Input: part model. Units: mm. Frame: model coordinates. Face numbers are marked on the shaded views. A direction names the side the tool comes from. Give positions to 0.01 mm unless a question says otherwise; leave off trailing zeros. Loops run counter-clockwise (first coordinate to the right, second up) from the corner with the lowest first, then second, coordinate; pieces in that order, holes last. Notation, with made-up numbers: M 86.5,-11.5 L 113.5,-11.5 A12 cw 113.5,6.5 Z; hole C 88,18.25 d7. An arc over 180 degrees is marked long. Use a Markdown table: item, result. Add a question column.
from build123d import *

# Parameters (mm, degrees)
F0_W     = 50
F0_H     = 1.4
F0_H_2   = 9.33334
F0_H_3   = 9.33333
F0_W_2   = 2
F1_DEPTH = 2
F2_DEPTH = 12.2
F3_DEPTH = 4.4


with BuildPart() as f1:
    # F0 (on Top) → F1 (new body)
    with BuildSketch(Plane.XY):
        with BuildLine():
            ThreePointArc((21.8201372772, -22.06666), (27.3605822843, -24.3541997855), (25.0540951786, -18.8216157258))
            Line((25.0540951786, -18.8216157258), (25.0540951786, -20.06666))
            Line((25.0540951786, -20.06666), (25.0540951786, -20.46666))
            ThreePointArc((25.0540951786, -20.46666), (26.1854660285, -20.9352891501), (26.6540951786, -22.06666))
            ThreePointArc((26.6540951786, -22.06666), (25.0540951786, -23.66666), (23.4540951786, -22.06666))
            Line((23.4540951786, -22.06666), (23.0540951786, -22.06666))
            Line((23.0540951786, -22.06666), (21.8201372772, -22.06666))
        make_face()
        with Locations((-1.9459048214, 0.7)):
            Rectangle(F0_W, F0_H)
        with BuildLine():
            Line((-26.9459048214, 12.73334), (-27.3459048214, 12.73334))
            ThreePointArc((-27.3459048214, 12.73334), (-27.8145339715, 11.6019691501), (-28.9459048214, 11.13334))
            Line((-28.9459048214, 11.13334), (-28.9459048214, 10.73334))
            Line((-28.9459048214, 10.73334), (-26.9459048214, 10.73334))
            Line((-26.9459048214, 10.73334), (-26.9459048214, 12.73334))
        make_face()
        with BuildLine():
            Line((-26.9459048214, -22.06666), (-26.9459048214, -20.06666))
            Line((-26.9459048214, -20.06666), (-28.9459048214, -20.06666))
            Line((-28.9459048214, -20.06666), (-28.9459048214, -20.46666))
            ThreePointArc((-28.9459048214, -20.46666), (-27.8145339715, -20.9352891501), (-27.3459048214, -22.06666))
            Line((-27.3459048214, -22.06666), (-26.9459048214, -22.06666))
        make_face()
        with BuildLine():
            Line((23.0540951786, 12.73334), (23.0540951786, 10.73334))
            Line((23.0540951786, 10.73334), (25.0540951786, 10.73334))
            Line((25.0540951786, 10.73334), (25.0540951786, 11.1939641141))
            ThreePointArc((25.0540951786, 11.1939641141), (23.9822411075, 11.6614859288), (23.5147192927, 12.73334))
            Line((23.5147192927, 12.73334), (23.0540951786, 12.73334))
        make_face()
        with Locations((-1.9459048214, 6.06667)):
            Rectangle(F0_W, F0_H_2)
        Polygon((-26.9459048214, 10.73334), (-28.9459048214, 10.73334), (-28.9459048214, 9.7067784518), (-28.9459048214, 1.4), (-26.9459048214, 1.4), align=None)
        with Locations((-1.9459048214, -4.666665)):
            Rectangle(F0_W, F0_H_3)
        with BuildLine():
            ThreePointArc((25.0540951786, 9.4220731407), (27.3739572404, 15.169460212), (21.67487517, 12.73334))
            Line((21.67487517, 12.73334), (23.0540951786, 12.73334))
            Line((23.0540951786, 12.73334), (23.5147192927, 12.73334))
            ThreePointArc((23.5147192927, 12.73334), (25.0838484178, 14.3925799209), (26.7136119574, 12.7928567787))
            ThreePointArc((26.7136119574, 12.7928567787), (26.2237410386, 11.6406356962), (25.0540951786, 11.1939641141))
            Line((25.0540951786, 11.1939641141), (25.0540951786, 10.73334))
            Line((25.0540951786, 10.73334), (25.0540951786, 9.4220731407))
        make_face()
        with Locations((24.0540951786, -10.03333)):
            Rectangle(F0_W_2, F0_H)
        with BuildLine():
            ThreePointArc((-28.9459048214, 11.13334), (-30.0772756713, 13.8647108499), (-27.3459048214, 12.73334))
            Line((-27.3459048214, 12.73334), (-26.9459048214, 12.73334))
            Line((-26.9459048214, 12.73334), (-26.0620750487, 12.73334))
            ThreePointArc((-26.0620750487, 12.73334), (-31.1388180647, 14.6834699023), (-28.9459048214, 9.7067784518))
            Line((-28.9459048214, 9.7067784518), (-28.9459048214, 10.73334))
            Line((-28.9459048214, 10.73334), (-28.9459048214, 11.13334))
        make_face()
        with BuildLine():
            Line((-28.9459048214, -20.06666), (-28.9459048214, -19.0631560981))
            ThreePointArc((-28.9459048214, -19.0631560981), (-31.0781165452, -24.1453706629), (-25.9737856686, -22.06666))
            Line((-25.9737856686, -22.06666), (-26.9459048214, -22.06666))
            Line((-26.9459048214, -22.06666), (-27.3459048214, -22.06666))
            ThreePointArc((-27.3459048214, -22.06666), (-30.0772756713, -23.1980308499), (-28.9459048214, -20.46666))
            Line((-28.9459048214, -20.46666), (-28.9459048214, -20.06666))
        make_face()
        Polygon((-26.0620750487, 12.73334), (-26.9459048214, 12.73334), (-26.9459048214, 10.73334), (23.0540951786, 10.73334), (23.0540951786, 12.73334), (21.67487517, 12.73334), align=None)
        Polygon((23.0540951786, -20.06666), (-26.9459048214, -20.06666), (-26.9459048214, -22.06666), (-25.9737856686, -22.06666), (21.8201372772, -22.06666), (23.0540951786, -22.06666), align=None)
        with Locations((-27.9459048214, 0.7)):
            Rectangle(F0_W_2, F0_H)
        with Locations((24.0540951786, 0.7)):
            Rectangle(F0_W_2, F0_H)
        with Locations((-27.9459048214, -4.666665)):
            Rectangle(F0_W_2, F0_H_3)
        with Locations((24.0540951786, -4.666665)):
            Rectangle(F0_W_2, F0_H_3)
        with Locations((-27.9459048214, -10.03333)):
            Rectangle(F0_W_2, F0_H)
        with Locations((-1.9459048214, -15.399995)):
            Rectangle(F0_W, F0_H_3)
        with BuildLine():
            Line((25.0540951786, -20.06666), (23.0540951786, -20.06666))
            Line((23.0540951786, -20.06666), (23.0540951786, -22.06666))
            Line((23.0540951786, -22.06666), (23.4540951786, -22.06666))
            ThreePointArc((23.4540951786, -22.06666), (23.9227243287, -20.9352891501), (25.0540951786, -20.46666))
            Line((25.0540951786, -20.46666), (25.0540951786, -20.06666))
        make_face()
        Polygon((-26.9459048214, -20.06666), (-26.9459048214, -10.73333), (-28.9459048214, -10.73333), (-28.9459048214, -19.0631560981), (-28.9459048214, -20.06666), align=None)
        Polygon((25.0540951786, 10.73334), (23.0540951786, 10.73334), (23.0540951786, 1.4), (25.0540951786, 1.4), (25.0540951786, 9.4220731407), align=None)
        with Locations((-1.9459048214, -10.03333)):
            Rectangle(F0_W, F0_H)
        Polygon((25.0540951786, -10.73333), (23.0540951786, -10.73333), (23.0540951786, -20.06666), (25.0540951786, -20.06666), (25.0540951786, -18.8216157258), align=None)
    extrude(amount=F1_DEPTH)

    # F0 (on Top) → F2 (join)
    with BuildSketch(Plane.XY):
        Polygon((-26.0620750487, 12.73334), (-26.9459048214, 12.73334), (-26.9459048214, 10.73334), (23.0540951786, 10.73334), (23.0540951786, 12.73334), (21.67487517, 12.73334), align=None)
        Polygon((-26.9459048214, 10.73334), (-28.9459048214, 10.73334), (-28.9459048214, 9.7067784518), (-28.9459048214, 1.4), (-26.9459048214, 1.4), align=None)
        with Locations((-27.9459048214, -4.666665)):
            Rectangle(F0_W_2, F0_H_3)
        Polygon((-26.9459048214, -20.06666), (-26.9459048214, -10.73333), (-28.9459048214, -10.73333), (-28.9459048214, -19.0631560981), (-28.9459048214, -20.06666), align=None)
        Polygon((23.0540951786, -20.06666), (-26.9459048214, -20.06666), (-26.9459048214, -22.06666), (-25.9737856686, -22.06666), (21.8201372772, -22.06666), (23.0540951786, -22.06666), align=None)
        Polygon((25.0540951786, -10.73333), (23.0540951786, -10.73333), (23.0540951786, -20.06666), (25.0540951786, -20.06666), (25.0540951786, -18.8216157258), align=None)
        with Locations((24.0540951786, -4.666665)):
            Rectangle(F0_W_2, F0_H_3)
        with Locations((24.0540951786, -10.03333)):
            Rectangle(F0_W_2, F0_H)
        with Locations((-27.9459048214, -10.03333)):
            Rectangle(F0_W_2, F0_H)
        Polygon((25.0540951786, 10.73334), (23.0540951786, 10.73334), (23.0540951786, 1.4), (25.0540951786, 1.4), (25.0540951786, 9.4220731407), align=None)
        with Locations((24.0540951786, 0.7)):
            Rectangle(F0_W_2, F0_H)
        with Locations((-27.9459048214, 0.7)):
            Rectangle(F0_W_2, F0_H)
        with BuildLine():
            ThreePointArc((25.0540951786, 9.4220731407), (27.3739572404, 15.169460212), (21.67487517, 12.73334))
            Line((21.67487517, 12.73334), (23.0540951786, 12.73334))
            Line((23.0540951786, 12.73334), (23.5147192927, 12.73334))
            ThreePointArc((23.5147192927, 12.73334), (25.0838484178, 14.3925799209), (26.7136119574, 12.7928567787))
            ThreePointArc((26.7136119574, 12.7928567787), (26.2237410386, 11.6406356962), (25.0540951786, 11.1939641141))
            Line((25.0540951786, 11.1939641141), (25.0540951786, 10.73334))
            Line((25.0540951786, 10.73334), (25.0540951786, 9.4220731407))
        make_face()
        with BuildLine():
            ThreePointArc((21.8201372772, -22.06666), (27.3605822843, -24.3541997855), (25.0540951786, -18.8216157258))
            Line((25.0540951786, -18.8216157258), (25.0540951786, -20.06666))
            Line((25.0540951786, -20.06666), (25.0540951786, -20.46666))
            ThreePointArc((25.0540951786, -20.46666), (26.1854660285, -20.9352891501), (26.6540951786, -22.06666))
            ThreePointArc((26.6540951786, -22.06666), (25.0540951786, -23.66666), (23.4540951786, -22.06666))
            Line((23.4540951786, -22.06666), (23.0540951786, -22.06666))
            Line((23.0540951786, -22.06666), (21.8201372772, -22.06666))
        make_face()
        with BuildLine():
            Line((25.0540951786, -20.06666), (23.0540951786, -20.06666))
            Line((23.0540951786, -20.06666), (23.0540951786, -22.06666))
            Line((23.0540951786, -22.06666), (23.4540951786, -22.06666))
            ThreePointArc((23.4540951786, -22.06666), (23.9227243287, -20.9352891501), (25.0540951786, -20.46666))
            Line((25.0540951786, -20.46666), (25.0540951786, -20.06666))
        make_face()
        with BuildLine():
            Line((23.0540951786, 12.73334), (23.0540951786, 10.73334))
            Line((23.0540951786, 10.73334), (25.0540951786, 10.73334))
            Line((25.0540951786, 10.73334), (25.0540951786, 11.1939641141))
            ThreePointArc((25.0540951786, 11.1939641141), (23.9822411075, 11.6614859288), (23.5147192927, 12.73334))
            Line((23.5147192927, 12.73334), (23.0540951786, 12.73334))
        make_face()
        with BuildLine():
            Line((-26.9459048214, -22.06666), (-26.9459048214, -20.06666))
            Line((-26.9459048214, -20.06666), (-28.9459048214, -20.06666))
            Line((-28.9459048214, -20.06666), (-28.9459048214, -20.46666))
            ThreePointArc((-28.9459048214, -20.46666), (-27.8145339715, -20.9352891501), (-27.3459048214, -22.06666))
            Line((-27.3459048214, -22.06666), (-26.9459048214, -22.06666))
        make_face()
        with BuildLine():
            Line((-28.9459048214, -20.06666), (-28.9459048214, -19.0631560981))
            ThreePointArc((-28.9459048214, -19.0631560981), (-31.0781165452, -24.1453706629), (-25.9737856686, -22.06666))
            Line((-25.9737856686, -22.06666), (-26.9459048214, -22.06666))
            Line((-26.9459048214, -22.06666), (-27.3459048214, -22.06666))
            ThreePointArc((-27.3459048214, -22.06666), (-30.0772756713, -23.1980308499), (-28.9459048214, -20.46666))
            Line((-28.9459048214, -20.46666), (-28.9459048214, -20.06666))
        make_face()
        with BuildLine():
            ThreePointArc((-28.9459048214, 11.13334), (-30.0772756713, 13.8647108499), (-27.3459048214, 12.73334))
            Line((-27.3459048214, 12.73334), (-26.9459048214, 12.73334))
            Line((-26.9459048214, 12.73334), (-26.0620750487, 12.73334))
            ThreePointArc((-26.0620750487, 12.73334), (-31.1388180647, 14.6834699023), (-28.9459048214, 9.7067784518))
            Line((-28.9459048214, 9.7067784518), (-28.9459048214, 10.73334))
            Line((-28.9459048214, 10.73334), (-28.9459048214, 11.13334))
        make_face()
        with BuildLine():
            Line((-26.9459048214, 12.73334), (-27.3459048214, 12.73334))
            ThreePointArc((-27.3459048214, 12.73334), (-27.8145339715, 11.6019691501), (-28.9459048214, 11.13334))
            Line((-28.9459048214, 11.13334), (-28.9459048214, 10.73334))
            Line((-28.9459048214, 10.73334), (-26.9459048214, 10.73334))
            Line((-26.9459048214, 10.73334), (-26.9459048214, 12.73334))
        make_face()
    extrude(amount=F2_DEPTH)

    # F0 (on Top) → F3 (join)
    with BuildSketch(Plane.XY):
        with Locations((-1.9459048214, 0.7)):
            Rectangle(F0_W, F0_H)
        with Locations((-1.9459048214, -10.03333)):
            Rectangle(F0_W, F0_H)
    extrude(amount=F3_DEPTH)


solid = f1.part
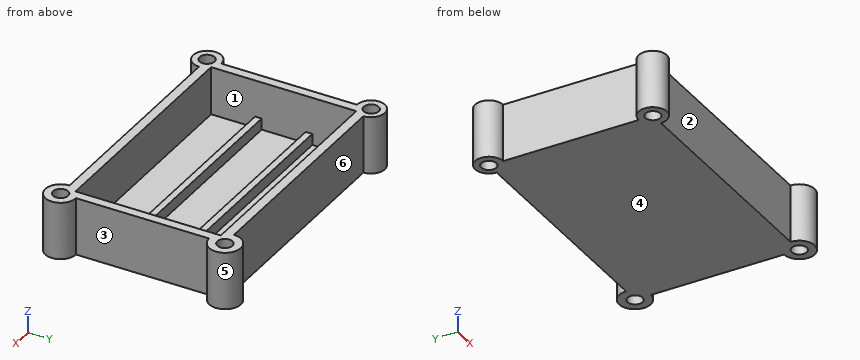
1) Section query D-D, the plane y = -15.5. Return the cut outline in (x, z), and give its area (3 significant figures).
2) Reachability of the marked faces 1, 2 and 3 from +Z, -Z, +X, -X, +Y, -Y: full face, straight path, thin tool, end or side. Return the list, or none.
3) Pull-direction query (Y, two-part tool) for the marked faces 4, 5 and 6; classes: pulls with the +Y half, pulls with the -Y half, needs draft (parallel to the pull), parting line crosses it, or undercut.
4) Ray query, line 1 (Y direction, x = -8.5, z = 2.75); line 2 (Y direction, x = 25, z = 7.75); line 3 (X direction, y = 6, z = 11.75). Return the intervals inside material, ascending. Write a range as [from, to].
5) Contact query for flat-ended pins moving along their axis: P1, Ø5, axis at x = -2.5, z = 3.5, coming from the -Y side; P2, Ø1.1, axis at x = -12.5, y = 1, coming from the +Z side; P3, Ø1.5, axis at y = -21, z = 10.5, coming from the +X side. Output: stop coordinate, or through.
6) Section query B-B, the plane z = 9.75. Return the cut outline in (x, y), and give its area (3 significant figures).
7) Section query C-C, the plane x = 0. Return the cut outline in (y, z), and give its area (3 significant figures).
8) Section query A-A, the plane y = 12. Return the cut outline in (x, z).
Entries:
| question | item | result |
|---|---|---|
| 1 | outline | M -28.95,0 L 25.05,0 L 25.05,12.2 L 23.05,12.2 L 23.05,2 L -26.95,2 L -26.95,12.2 L -28.95,12.2 Z |
| 1 | area | 149 mm² |
| 2 | face 1 | +Z |
| 2 | face 2 | +Z, -Z, -Y |
| 2 | face 3 | +Z, -Z, +X |
| 3 | face 4 | needs draft |
| 3 | face 5 | undercut |
| 3 | face 6 | pulls with the +Y half |
| 4 | line 1 | y = [-22.07, -20.07], [-10.73, -9.33], [0, 1.4], [10.73, 12.73] |
| 4 | line 2 | y = [-25.31, -23.67], [-20.47, 11.2], [14.39, 16.13] |
| 4 | line 3 | x = [-28.95, -26.95], [23.05, 25.05] |
| 5 | P1 | stops at y = -22.07 |
| 5 | P2 | stops at z = 4.4 |
| 5 | P3 | stops at x = 28.29 |
| 6 | outline | M -28.95,-19.06 A2.98 ccw long -25.97,-22.07 L 21.82,-22.07 A3.24 ccw long 25.05,-18.82 L 25.05,9.42 A3.35 ccw long 21.67,12.73 L -26.06,12.73 A2.95 ccw long -28.95,9.71 Z; hole C -28.95,-22.07 d3.2; hole C -28.95,12.73 d3.2; hole M -26.95,-20.07 L 23.05,-20.07 L 23.05,10.73 L -26.95,10.73 Z; hole C 25.05,-22.07 d3.2; hole C 25.11,12.79 d3.2 |
| 6 | area | 400 mm² |
| 7 | outline | M -22.07,0 L 12.73,0 L 12.73,12.2 L 10.73,12.2 L 10.73,2 L 1.4,2 L 1.4,4.4 L 0,4.4 L 0,2 L -9.33,2 L -9.33,4.4 L -10.73,4.4 L -10.73,2 L -20.07,2 L -20.07,12.2 L -22.07,12.2 Z |
| 7 | area | 117 mm² |
| 8 | outline | M -31.88,0 L -30.37,0 L -30.37,12.2 L -31.88,12.2 Z; M -27.52,0 L 23.72,0 L 23.72,12.2 L -27.52,12.2 Z; M 26.5,0 L 28.29,0 L 28.29,12.2 L 26.5,12.2 Z |
